Autodesk Inventor part; units mm, degrees
ref_plane "YZ Plane" through (0, 0, 0) normal (1, 0, 0) x (0, 1, 0)
ref_plane "XZ Plane" through (0, 0, 0) normal (0, 1, 0) x (-1, 0, 0)
ref_plane "XY Plane" through (0, 0, 0) normal (0, 0, 1) x (1, 0, 0)
sketch "Sketch1" plane through (0, 0, 0) normal (0, 0, 1) x (1, 0, 0)
  line L0 (0, 0) -> (62, 0)
  line L1 (62, 0) -> (62, 40)
  line L2 (62, 40) -> (0, 40)
  line L3 (0, 40) -> (0, 0)
  line L4 (20, 40) -> (62, 40) construction
  line L5 (62, 40) -> (62, -2) construction
  line L6 (62, -2) -> (20, -2) construction
  line L7 (20, -2) -> (20, 40) construction
  line L8 (25.5, 34.5) -> (56.5, 34.5) construction
  line L9 (56.5, 34.5) -> (56.5, 3.5) construction
  line L10 (56.5, 3.5) -> (25.5, 3.5) construction
  line L11 (25.5, 3.5) -> (25.5, 34.5) construction
  point P0 (25.5, 19)
  point P1 (20, 19)
  point P2 (41, 34.5)
  point P3 (41, 40)
  point P4 (41, 19)
  point P5 (10, 30)
  point P6 (10, 10)
  dimension "d0" = 40
  dimension "d1" = 62
  dimension "d2" = 42
  dimension "d3" = 42
  dimension "d4" = 31
  dimension "d5" = 31
  dimension "d22" = 10
  dimension "d23" = 10
  dimension "d24" = 10
extrude "Extrusion1" add sketch "Sketch1" against normal blind 6.35
hole "Hole1" at (25.5, 34.5, 0) at (56.5, 34.5, 0) at (56.5, 3.5, 0) at (25.5, 3.5, 0) at (10, 30, 0) at (10, 10, 0) direction (0, 0, -1) diameter 3.2 end through all counterbore diameter 6.2 counterbore depth 3
hole "Hole2" at (41, 19, 0) direction (0, 0, -1) diameter 25 end through all
properties part number "Y Motor Mount"
Check sheet for the modelled part. Datum: model origin and axes. Units: mm. A direction names the side the tool comes from. Round coordinates to 2 decimals unless told otherwise and drop trailing zeros. Order: outer loops, then holes, each group sorted by start corner. A loop starts at its lowest first (then second) coordinate and runs counter-clockwise, first axis right, second up. Notation, with made-up numbers: (-26.75, 31.25) -> (29.25, 31.25) arc R20 ccw to (29.25, 59.25) -> close; hole circle Ø1 at (-38, -31.5). An arc over 180 degrees is marked (long way). One line per item, written item: value. Start each with the question number.
Q1. Cross-section at B-B (y = 19). Record the boundary of the cut face in (x, z).
Q2. Cross-section at A-A (x = 56.5). Record the boundary of the cut face in (y, z).
Q3. Cross-section at C-C (z = -5.5). Record the boundary of the cut face in (x, y).
Q4. Set-up check for faces 1 (the face through (55.15, 2.64, -4.7)), 2 (the face through (53.426, 3.904, -1.521)): record each of +Z, -Z, +X, -X, +Y, -Y from which the full face is reachable in a straight line by a thin tool's end or side.
Q5. Mould release check, pull along Y, two halves, no side actions. Record for faces 3 (the face through (31, 0, -3)), 4 (the face through (23.914, 3.708, -4.698)), 5 (the face through (24, 20, 0)), 6 (the face through (27, 2, -3)): pulls with the +Y half, pulls with the -Y half, needs draft (parallel to the pull), parting line crosses it, or undercut.
Q6. Gauge pin test, flat ends, axial feed: pin 1 Ø1 at (x, y) = (40, 29) entering from +Z; pin 2 Ø1.9 at (x, y) = (9, 10) entering from +Z. Record the tip position at first contact, or that the pin passes through.
Q7. Thickness scan on line 1 (Y direction, x = 25.5, z = -5.45); line 2 (Y direction, x = 10, z = -4.65); line 3 (X direction, y = 34.5, z = -0.7). Record the ranges inside material, lowest first.
Q8. Cross-section at D-D (y = 34.5). Record the boundary of the cut face in (x, z), and give its area (3 significant figures).
Completed:
1. outline: (0, -6.35) -> (28.5, -6.35) -> (28.5, 0) -> (0, 0) -> close; (53.5, -6.35) -> (62, -6.35) -> (62, 0) -> (53.5, 0) -> close
2. outline: (0, -6.35) -> (1.9, -6.35) -> (1.9, -3) -> (0.4, -3) -> (0.4, 0) -> (0, 0) -> close; (5.1, -6.35) -> (32.9, -6.35) -> (32.9, -3) -> (31.4, -3) -> (31.4, 0) -> (6.6, 0) -> (6.6, -3) -> (5.1, -3) -> close; (36.1, -6.35) -> (40, -6.35) -> (40, 0) -> (37.6, 0) -> (37.6, -3) -> (36.1, -3) -> close
3. outline: (0, 0) -> (62, 0) -> (62, 40) -> (0, 40) -> close; hole circle Ø3.2 at (10, 10); hole circle Ø3.2 at (10, 30); hole circle Ø3.2 at (25.5, 3.5); hole circle Ø3.2 at (25.5, 34.5); hole circle Ø25 at (41, 19); hole circle Ø3.2 at (56.5, 3.5); hole circle Ø3.2 at (56.5, 34.5)
4. face 1: +Z, -Z
4. face 2: +Z
5. face 3: pulls with the -Y half
5. face 4: undercut
5. face 5: needs draft
5. face 6: undercut
6. pin 1: passes through
6. pin 2: stops at z = -3
7. line 1: y = 0 to 1.9, 5.1 to 32.9, 36.1 to 40
7. line 2: y = 0 to 8.4, 11.6 to 28.4, 31.6 to 40
7. line 3: x = 0 to 22.4, 28.6 to 53.4, 59.6 to 62
8. outline: (0, -6.35) -> (23.9, -6.35) -> (23.9, -3) -> (22.4, -3) -> (22.4, 0) -> (0, 0) -> close; (27.1, -6.35) -> (54.9, -6.35) -> (54.9, -3) -> (53.4, -3) -> (53.4, 0) -> (28.6, 0) -> (28.6, -3) -> (27.1, -3) -> close; (58.1, -6.35) -> (62, -6.35) -> (62, 0) -> (59.6, 0) -> (59.6, -3) -> (58.1, -3) -> close
8. area: 335 mm²
